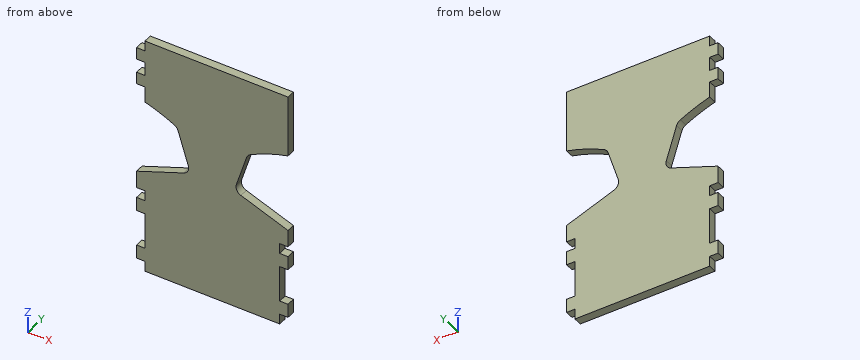
```python
from build123d import *

# Parameters (mm, degrees)
BOSS_EXTRUDE1_DEPTH = 3.048


with BuildPart() as part:
    # Sketch1 → Boss-Extrude1 (new, symmetric)
    with BuildSketch(Plane(origin=(0, 0, 0), x_dir=(1, 0, 0), z_dir=(0, 1, 0))):
        with BuildLine():
            Line((-49.53, 45.72), (49.53, 45.72))
            Line((49.53, 45.72), (49.53, 38.1))
            Line((49.53, 38.1), (55.626, 38.1))
            Line((55.626, 38.1), (55.626, 27.94))
            Line((55.626, 27.94), (49.53, 27.94))
            Line((49.53, 27.94), (49.53, 1.208143374))
            Line((49.53, 1.208143374), (55.626, 1.208143374))
            Line((55.626, 1.208143374), (55.626, -8.951856626))
            Line((55.626, -8.951856626), (49.53, -8.951856626))
            Line((49.53, -8.951856626), (49.53, -16.571856626))
            Line((49.53, -16.571856626), (55.626, -16.571856626))
            Line((55.626, -16.571856626), (55.626, -29.271856626))
            Line((55.626, -29.271856626), (21.019827136, -42.136821893))
            ThreePointArc((21.019827136, -42.136821893), (17.95098831, -44.911778638), (17.631953735, -49.036869377))
            Line((17.631953735, -49.036869377), (25.187729856, -73.287029113))
            ThreePointArc((25.187729856, -73.287029113), (26.234780075, -75.207903536), (27.939063878, -76.579577488))
            ThreePointArc((27.939063878, -76.579577488), (41.468907088, -82.632484358), (55.626, -87.022365809))
            Line((55.626, -87.022365809), (55.626, -132.617292876))
            Line((55.626, -132.617292876), (-49.53, -132.617292876))
            Line((-49.53, -132.617292876), (-49.53, -124.997292876))
            Line((-49.53, -124.997292876), (-55.626, -124.997292876))
            Line((-55.626, -124.997292876), (-55.626, -116.107292876))
            Line((-55.626, -116.107292876), (-49.53, -116.107292876))
            Line((-49.53, -116.107292876), (-49.53, -105.947292876))
            Line((-49.53, -105.947292876), (-55.626, -105.947292876))
            Line((-55.626, -105.947292876), (-55.626, -97.057292876))
            Line((-55.626, -97.057292876), (-49.53, -97.057292876))
            Line((-49.53, -97.057292876), (-49.53, -85.359826344))
            ThreePointArc((-49.53, -85.359826344), (-38.527111219, -81.479756652), (-27.939063878, -76.579577488))
            ThreePointArc((-27.939063878, -76.579577488), (-26.234780075, -75.207903536), (-25.187729856, -73.287029113))
            Line((-25.187729856, -73.287029113), (-17.631953735, -49.036869377))
            ThreePointArc((-17.631953735, -49.036869377), (-17.95098831, -44.911778638), (-21.019827136, -42.136821893))
            Line((-21.019827136, -42.136821893), (-55.626, -29.271856626))
            Line((-55.626, -29.271856626), (-55.626, -16.571856626))
            Line((-55.626, -16.571856626), (-49.53, -16.571856626))
            Line((-49.53, -16.571856626), (-49.53, -8.951856626))
            Line((-49.53, -8.951856626), (-55.626, -8.951856626))
            Line((-55.626, -8.951856626), (-55.626, 1.208143374))
            Line((-55.626, 1.208143374), (-49.53, 1.208143374))
            Line((-49.53, 1.208143374), (-49.53, 27.94))
            Line((-49.53, 27.94), (-55.626, 27.94))
            Line((-55.626, 27.94), (-55.626, 38.1))
            Line((-55.626, 38.1), (-49.53, 38.1))
            Line((-49.53, 38.1), (-49.53, 45.72))
        make_face()
    extrude(amount=BOSS_EXTRUDE1_DEPTH, both=True)


solid = part.part
```
Build history of the part. All positions in model axes, mm. Give positions to 0.01 mm unless a question says otherwise; leave off trailing zeros. Loops run counter-clockwise (first coordinate to the right, second up) from the corner with the lowest first, then second, coordinate; pieces in that order, holes last.
1) Drop flat-ended pins along their axis: P1, Ø3, axis at x = -53.5, y = 0, coming from the -Z side; P2, Ø1.8, axis at y = -1, z = 127.5, coming from the -X side; P3, Ø1.8, axis at y = 1.5, z = -43, coming from the +X side. Give the stop position or say it passes through.
Values follow:
P1: stops at z = -38.1
P2: stops at x = -49.53
P3: stops at x = 49.53
2) Band-saw the part on A-A on x = 44. List the corners of the cut face in (y, z).
Values follow:
outline: (-3.05, -45.72) - (3.05, -45.72) - (3.05, 33.59) - (-3.05, 33.59) - close; (-3.05, 83.56) - (3.05, 83.56) - (3.05, 132.62) - (-3.05, 132.62) - close
3) Probe line 1 along X through (y, z) = (-0.25, -18); line 2 along Z through (x, y) = (-36.5, 2.5); line 3 along Z through (x, y) = (32.5, -0.25). List the from-to ranges inside material, lowest first.
Values follow:
line 1: x = -49.53 to 49.53
line 2: z = -45.72 to 36.38, 80.63 to 132.62
line 3: z = -45.72 to 37.87, 78.84 to 132.62
4) Band-saw the part on B-B on z = 110. List the corners of the cut face in (x, y), then the cut area to 3 significant figures.
Values follow:
outline: (-49.53, -3.05) - (55.63, -3.05) - (55.63, 3.05) - (-49.53, 3.05) - close
area: 641 mm2
5) Band-saw the part on C-C on z = -12. List the corners of the cut face in (x, y), then the cut area to 3 significant figures.
Values follow:
outline: (-49.53, -3.05) - (49.53, -3.05) - (49.53, 3.05) - (-49.53, 3.05) - close
area: 604 mm2
